from build123d import *
from build123d import SkipClean  # not in build123d's __all__

# Parameters (mm, degrees)
F0_R     = 75
F0_R_2   = 10
F1_DEPTH = 50
F6_DEPTH = 15


# Not quite as in the source:
# - a pattern or mirror of a feature is missing from the dataset's text; its kind, count and spacing are read off the source's solid


with BuildPart() as f1:
    # F0 (on Front) → F1 (new body)
    with BuildSketch(Plane.XZ):
        Circle(F0_R)
        with BuildLine():
            ThreePointArc((-57.5027136201, -17.1300299569), (-39.4445240133, -0.6421875508), (-15, 0))
            ThreePointArc((-15, 0), (-13.6930639376, -6.123724357), (-10, -11.1803398875))
            ThreePointArc((-10, -11.1803398875), (-11.2445250944, -37.3888406037), (2.1300299569, -59.9621795166))
            ThreePointArc((2.1300299569, -59.9621795166), (-35.0025968036, -48.7321066342), (-57.5027136201, -17.1300299569))
        make_face(mode=Mode.SUBTRACT)
        with BuildLine():
            ThreePointArc((17.1300299569, -57.5027136201), (0.6421875508, -39.4445240133), (0, -15))
            ThreePointArc((0, -15), (6.123724357, -13.6930639376), (11.1803398875, -10))
            ThreePointArc((11.1803398875, -10), (37.3888406037, -11.2445250944), (59.9621795166, 2.1300299569))
            ThreePointArc((59.9621795166, 2.1300299569), (48.7321066342, -35.0025968036), (17.1300299569, -57.5027136201))
        make_face(mode=Mode.SUBTRACT)
        with BuildLine():
            ThreePointArc((-59.9621795166, -2.1300299569), (-48.7321066342, 35.0025968036), (-17.1300299569, 57.5027136201))
            ThreePointArc((-17.1300299569, 57.5027136201), (-0.6421875508, 39.4445240133), (0, 15))
            ThreePointArc((0, 15), (-6.123724357, 13.6930639376), (-11.1803398875, 10))
            ThreePointArc((-11.1803398875, 10), (-37.3888406037, 11.2445250944), (-59.9621795166, -2.1300299569))
        make_face(mode=Mode.SUBTRACT)
        Circle(F0_R_2, mode=Mode.SUBTRACT)
        with BuildLine():
            ThreePointArc((15, 0), (13.6930639376, 6.123724357), (10, 11.1803398875))
            ThreePointArc((10, 11.1803398875), (11.2445250944, 37.3888406037), (-2.1300299569, 59.9621795166))
            ThreePointArc((-2.1300299569, 59.9621795166), (35.0025968036, 48.7321066342), (57.5027136201, 17.1300299569))
            ThreePointArc((57.5027136201, 17.1300299569), (39.4445240133, 0.6421875508), (15, 0))
        make_face(mode=Mode.SUBTRACT)
    extrude(amount=F1_DEPTH)

    # F2 (on Right) → F3 (revolve)
    with BuildSketch(Plane.YZ):
        with BuildLine():
            Line((-50, 75), (0, 75))
            ThreePointArc((0, 75), (-25, 88.4168760482), (-50, 75))
        make_face()
    revolve(axis=Axis((0, -25, 0), (0, -1, 0)))

    # F5 (on face) → F6 (cut)
    with BuildSketch(Plane.XZ.offset(50)):
        with BuildLine():
            ThreePointArc((-17.1300299569, 57.5027136201), (-0.6421875508, 39.4445240133), (0, 15))
            ThreePointArc((0, 15), (5.3523313466, 14.0125853844), (10, 11.1803398875))
            ThreePointArc((10, 11.1803398875), (11.2445250944, 37.3888406037), (-2.1300299569, 59.9621795166))
            ThreePointArc((-2.1300299569, 59.9621795166), (-9.7082295036, 59.2093766215), (-17.1300299569, 57.5027136201))
        make_face()
        with BuildLine():
            ThreePointArc((57.5027136201, 17.1300299569), (39.4445240133, 0.6421875508), (15, 0))
            ThreePointArc((15, 0), (14.0125853844, -5.3523313466), (11.1803398875, -10))
            ThreePointArc((11.1803398875, -10), (37.3888406037, -11.2445250944), (59.9621795166, 2.1300299569))
            ThreePointArc((59.9621795166, 2.1300299569), (59.2093766215, 9.7082295036), (57.5027136201, 17.1300299569))
        make_face()
        with BuildLine():
            ThreePointArc((17.1300299569, -57.5027136201), (0.6421875508, -39.4445240133), (0, -15))
            ThreePointArc((0, -15), (-5.3523313466, -14.0125853844), (-10, -11.1803398875))
            ThreePointArc((-10, -11.1803398875), (-11.2445250944, -37.3888406037), (2.1300299569, -59.9621795166))
            ThreePointArc((2.1300299569, -59.9621795166), (9.7082295036, -59.2093766215), (17.1300299569, -57.5027136201))
        make_face()
        with BuildLine():
            ThreePointArc((-57.5027136201, -17.1300299569), (-39.4445240133, -0.6421875508), (-15, 0))
            ThreePointArc((-15, 0), (-14.0125853844, 5.3523313466), (-11.1803398875, 10))
            ThreePointArc((-11.1803398875, 10), (-37.3888406037, 11.2445250944), (-59.9621795166, -2.1300299569))
            ThreePointArc((-59.9621795166, -2.1300299569), (-59.2093766215, -9.7082295036), (-57.5027136201, -17.1300299569))
        make_face()
    with SkipClean():  # cleaning this boolean's faces spoils the solid; the shape is the same uncleaned
        f6 = extrude(amount=-F6_DEPTH, mode=Mode.SUBTRACT)

    # F6_copies: F6 across plane
    with SkipClean():  # cleaning this boolean's faces spoils the solid; the shape is the same uncleaned
        add(f6.mirror(Plane.ZX.offset(-25)), clean=False, mode=Mode.SUBTRACT)


solid = f1.part
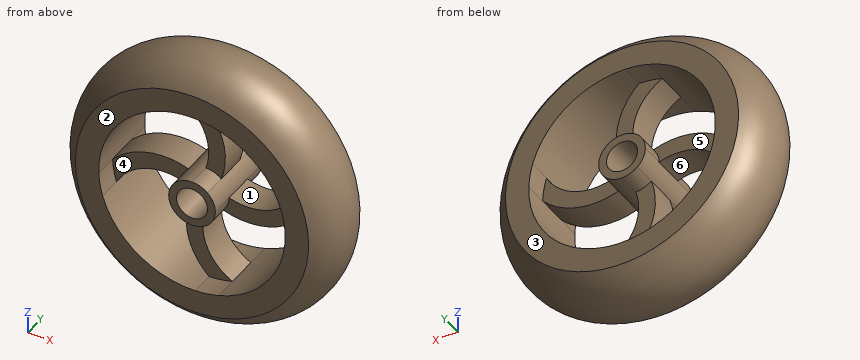
Can you work these out from the model? Positions are in its coordinate system, mm. Face numbers are marked on the shaded views. A direction names the side the tool comes from. Give positions to 0.01 mm unless a question says otherwise; leave off trailing zeros. Order: outer loops, then holes, each group sorted by start corner. A loop starts at its lowest first (then second) coordinate and runs counter-clockwise, first axis right, second up. Notation, with made-up numbers: M 15,-7.75 L 20,-7.75 A23 ccw 20,3.25 Z; hole C 38.25,65 d9. An arc over 180 degrees is marked long. Use one line per item in the form item = value. Start each with the question number.
Item 1: For the marked faces 3, 4, 5 and 6, which set-ups out of +Z, -Z, +X, -X, +Y, -Y let a thin tool reach every point of the face, with its end or its side?
Item 2: We'd pull the mould along Z, two halves only. Please class the marked faces 1 and 2: +Z half, -Z half, draft (parallel to the pull), parting line (faces both ways), or undercut.
Item 3: If I drill on line 1 along Z through (x, y) = (-30, -26.5); line 2 along X through (y, z) = (-23.5, 27.5); line 3 along X through (y, z) = (-5, 13.5), over which ranges is the centre line in solid material (lowest first)?
Item 4: If we section it at B-B (z = -50.5): State how many separate pieces and enclosed holes the cut face has, then the cut area to 3 significant figures.
Item 5: Will these pins go through, and if not, where does the flat tip stop? pin 1 Ø1 at (y, z) = (-9, -47.5) entering from -X; pin 2 Ø4 at (y, z) = (-18.5, -44.5) entering from -X; pin 3 Ø3 at (y, z) = (-6, -18) entering from -X; pin 4 Ø6 at (x, z) = (9, -4) entering from -Y.
Item 6: If we section it at A-A (y = -18): Write out the boundary of the cut face in (x, z).
Outcome:
q1.face_3 = +Z, -Z, +X, -X, +Y
q1.face_4 = -Y
q1.face_5 = +Y
q1.face_6 = +Y, -Y
q2.face_1 = undercut
q2.face_2 = draft
q3.line_1 = -83.13 to -51.96, 1.71 to 12.45, 51.96 to 83.13
q3.line_2 = -83.99 to -53.33, 1.88 to 12.58, 53.33 to 83.99
q3.line_3 = -79.64 to -58.46, -6.54 to 6.54, 58.46 to 79.64
q4.separate_pieces = 3
q4.enclosed_holes = 0
q4.area = 3,790 mm2
q5.pin_1 = -69.54
q5.pin_2 = -76.82
q5.pin_3 = -80.85
q5.pin_4 = -50
q6.outline = C 0,0 d175.18; hole M -59.96,-2.13 A45.7 cw -11.18,10 A15 cw 0,15 A35 ccw -17.13,57.5 A60 ccw Z; hole M -57.5,-17.13 A60 ccw 2.13,-59.96 A45.7 cw -10,-11.18 A15 cw -15,0 A35 ccw Z; hole C 0,0 d20; hole M -2.13,59.96 A45.7 cw 10,11.18 A15 cw 15,0 A35 ccw 57.5,17.13 A60 ccw Z; hole M 0,-15 A35 ccw 17.13,-57.5 A60 ccw 59.96,2.13 A45.7 cw 11.18,-10 A15 cw Z
